For this review, take the finished solid that the model builds, in its own axes (mm). Face numbers are marked on the shaded views. A direction names the side the tool comes from. Round coordinates to 2 decimals unless told otherwise and drop trailing zeros. Order: outer loops, then holes, each group sorted by start corner. A loop starts at its lowest first (then second) coordinate and runs counter-clockwise, first axis right, second up.
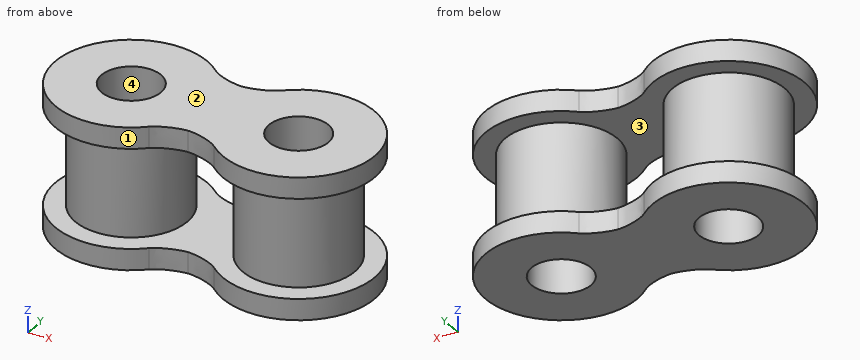
```python
from build123d import *

# Parameters (mm, degrees)
SKETCH_1_R        = 4.25
SKETCH_1_R_2      = 2.25
EXTRUDE_1_DEPTH   = 3.75
EXTRUDE_1_2_DEPTH = 3.75
SKETCH_2_R        = 5.75
SKETCH_2_R_2      = 4.25
SKETCH_2_R_3      = 2.25
EXTRUDE_3_DEPTH   = 1.6


with BuildPart() as part:
    # Sketch 1 → Extrude 1 (new body)
    with BuildSketch(Plane.XY):
        with Locations((-6.35, 0)):
            Circle(SKETCH_1_R)
        with Locations((-6.35, 0)):
            Circle(SKETCH_1_R_2, mode=Mode.SUBTRACT)
    extrude_1 = extrude(amount=EXTRUDE_1_DEPTH)



with BuildPart() as body_2:
    # Sketch 1 → Extrude 1 2 (new body)
    with BuildSketch(Plane.XY):
        with Locations(Location((6.35, 0, 0), (0, 0, 180))):
            Circle(SKETCH_1_R)
        with Locations(Location((6.35, 0, 0), (0, 0, 180))):
            Circle(SKETCH_1_R_2, mode=Mode.SUBTRACT)
    extrude_1_2 = extrude(amount=EXTRUDE_1_2_DEPTH)


with BuildPart() as part_1:
    add(part.part)

    add(body_2.part)  # Extrude 3 merges body 2
    # Sketch 2 → Extrude 3 (add)
    # profile 1 of 4: a face of its own
    with BuildSketch(Plane.XY.offset(3.75)):
        with Locations((-6.35, 0)):
            Circle(SKETCH_2_R)
        with Locations((-6.35, 0)):
            Circle(SKETCH_2_R_2, mode=Mode.SUBTRACT)
    # profile 2 of 4: a face of its own
    with BuildSketch(Plane.XY.offset(3.75)):
        with Locations((-6.35, 0)):
            Circle(SKETCH_2_R_2)
        with Locations((-6.35, 0)):
            Circle(SKETCH_2_R_3, mode=Mode.SUBTRACT)
    # profile 3 of 4: a face of its own
    with BuildSketch(Plane.XY.offset(3.75)):
        with BuildLine():
            ThreePointArc((-2.464522189, 4.238580208), (-1.086731177, 2.315275641), (-0.6, 0))
            ThreePointArc((-0.6, 0), (-1.086731177, -2.315275641), (-2.464522189, -4.238580208))
            add(Edge.make_bspline(
                [(-2.464522189, -4.238580208), (-1.801147303, -3.67793909), (-0.370790644, -3.34588107), (0, -3.386350938)],
                knots=[0, 0, 0, 0, 1, 1, 1, 1], degree=3))
            add(Edge.make_bspline(
                [(2.464522189, -4.238580208), (1.801147303, -3.67793909), (0.370790644, -3.34588107), (0, -3.386350938)],
                knots=[0, 0, 0, 0, 1, 1, 1, 1], degree=3))
            ThreePointArc((2.464522189, -4.238580208), (0.6, 0), (2.464522189, 4.238580208))
            add(Edge.make_bspline(
                [(2.464522189, 4.238580208), (1.801147303, 3.67793909), (0.370790644, 3.34588107), (0, 3.386350938)],
                knots=[0, 0, 0, 0, 1, 1, 1, 1], degree=3))
            add(Edge.make_bspline(
                [(-2.464522189, 4.238580208), (-1.801147303, 3.67793909), (-0.370790644, 3.34588107), (0, 3.386350938)],
                knots=[0, 0, 0, 0, 1, 1, 1, 1], degree=3))
        make_face()
    # profile 4 of 4: a face of its own
    with BuildSketch(Plane.XY.offset(3.75)):
        with Locations((6.35, 0)):
            Circle(SKETCH_2_R)
        with Locations(Location((6.35, 0, 0), (0, 0, 180))):
            Circle(SKETCH_2_R_3, mode=Mode.SUBTRACT)
    extrude_3 = extrude(amount=EXTRUDE_3_DEPTH)

    # Mirror 2: Extrude 1, Extrude 1 2, Extrude 3 across plane
    add(extrude_1.mirror(Plane(origin=(0, 0, 0), x_dir=(1, 0, 0), z_dir=(0, 0, -1))))
    add(extrude_1_2.mirror(Plane(origin=(0, 0, 0), x_dir=(1, 0, 0), z_dir=(0, 0, -1))))
    add(extrude_3.mirror(Plane(origin=(0, 0, 0), x_dir=(1, 0, 0), z_dir=(0, 0, -1))))


solid = part_1.part
```
Q1. Mouldability with a two-part tool opening along X and no side actions: class the marked faces 1 and 2 as +X half, -X half, draft (parallel to the pull), parting line (faces both ways), or undercut.
Q2. Wall thickness on line 1 (Z direction, x = -9.25, y = 3.5); line 2 (Y direction, x = -6.35, z = 2.5); line 3 (X direction, y = -1.5, z = -1.25): over which ranges is each line inside the solid? List them lowest first.
Q3. Take a section at B-B, the plane z = 3. State the section outline as (x, y) points.
Q4. Take a section at A-A, the plane x = 6.35. State the section outline as (y, z) points.
Q5. Take a section at D-D, the plane y = -4.5. State the section outline as (x, z) points, plus the area to 3 significant figures.
Q6. Clearance check with flat-ended pins moving along their axes: pin 1 (6 mm diameter, centred on y = 0.5, z = 0, fed in from +X); pin 2 (6 mm diameter, centred on x = 1.5, z = 0, fed in from +Y); pin 3 (1.5 mm diameter, centred on y = -4, z = 3.5, fed in from -X). State where each tip first meets the part, or that it passes through.
Q7. Take a section at C-C, the plane y = 1.75. State the section outline as (x, z) points, plus the area to 3 significant figures.
Q8. Tool access review of the marked faces 3 and 4: name each direction out of +Z, -Z, +X, -X, +Y, -Y from which nothing blocks a thin tool from reaching the whole face with its end or side.
Working result:
1. face 1: undercut
1. face 2: draft
2. line 1: z = -5.35 to -3.75, 3.75 to 5.35
2. line 2: y = -4.25 to -2.25, 2.25 to 4.25
2. line 3: x = -10.33 to -8.03, -4.67 to -2.37, 2.37 to 4.67, 8.03 to 10.33
3. outline: circle Ø8.5 at (-6.35, 0); circle Ø8.5 at (6.35, 0); hole circle Ø4.5 at (-6.35, 0); hole circle Ø4.5 at (6.35, 0)
4. outline: (-5.75, -5.35) - (-2.25, -5.35) - (-2.25, 5.35) - (-5.75, 5.35) - (-5.75, 3.75) - (-4.25, 3.75) - (-4.25, -3.75) - (-5.75, -3.75) - close; (2.25, -5.35) - (5.75, -5.35) - (5.75, -3.75) - (4.25, -3.75) - (4.25, 3.75) - (5.75, 3.75) - (5.75, 5.35) - (2.25, 5.35) - close
5. outline: (-9.93, -5.35) - (-2.77, -5.35) - (-2.77, -3.75) - (-9.93, -3.75) - close; (-9.93, 3.75) - (-2.77, 3.75) - (-2.77, 5.35) - (-9.93, 5.35) - close; (2.77, -5.35) - (9.93, -5.35) - (9.93, -3.75) - (2.77, -3.75) - close; (2.77, 3.75) - (9.93, 3.75) - (9.93, 5.35) - (2.77, 5.35) - close
5. area: 45.8 mm2
6. pin 1: stops at x = 10.6
6. pin 2: stops at y = 3.83
6. pin 3: stops at x = -11.06
7. outline: (-11.83, -5.35) - (-7.76, -5.35) - (-7.76, 5.35) - (-11.83, 5.35) - (-11.83, 3.75) - (-10.22, 3.75) - (-10.22, -3.75) - (-11.83, -3.75) - close; (-4.94, -5.35) - (4.94, -5.35) - (4.94, 5.35) - (-4.94, 5.35) - close; (7.76, -5.35) - (11.83, -5.35) - (11.83, -3.75) - (10.22, -3.75) - (10.22, 3.75) - (11.83, 3.75) - (11.83, 5.35) - (7.76, 5.35) - close; hole (-2.48, -3.75) - (2.48, -3.75) - (2.48, 3.75) - (-2.48, 3.75) - close
7. area: 131 mm2
8. face 3: none
8. face 4: +Z, -Z
